Geometry check sheet. Reference: the model listing, model coordinates, mm. A direction names the side the tool comes from. Coordinates: 2 decimals unless noted, no trailing zeros. Write each loop counter-clockwise with the first axis right and the second up, starting at its lowest first coordinate (ties: lowest second). Pieces come first, ordered by that corner, then holes. Notation, with made-up numbers: M 77,-33 L 91,-33 A23 cw 91,-6 Z; hole C -39.75,-7.75 d3. An arc over 180 degrees is marked long. Put each result on its own line as item: value. Start each with the question number.
1) Gauge pin test, flat ends, axial feed: pin 1 (3 mm diameter, centred on x = 110.5, z = -85.5, fed in from -Y); pin 2 (6.5 mm diameter, centred on x = 89, z = -85, fed in from -Y). Record the tip position at first contact, or that the pin passes through.
2) Cross-section at B-B on z = -85. Record the cut outline in (x, y).
3) Cross-section at A-A on x = 111. Record the cut outline in (y, z).
4) Mould release check, pull along X, two halves, no side actions. Record for faces 1 (the flat face through (99, 5, -100)), 2 (the flat face through (200, 5, -49)), 3 (the flat face through (108, 3.3, -85)): released by +X, released by -X, zero draft, split by the parting line, or undercut.
5) Set-up check for faces 4 (the flat face through (99, 0, -51)), 5 (the cylindrical face through (106.363, 1.627, -83.97)): record each of +Z, -Z, +X, -X, +Y, -Y from which the full face is reachable in a straight line by a thin tool's end or side.
6) Scan lines: line 1 along X through (y, z) = (5, -85); line 2 along X through (y, z) = (2.5, -85). Record each from-to range of solid material in increasing order.
from build123d import *

# Parameters (mm, degrees)
SKETCH_1_W                   = 200
SKETCH_1_H                   = 100
EXTRUDE_1_DEPTH              = 10
HOLE_WIZARD_M5_2_D           = 5.5
HOLE_WIZARD_M5_2_CBORE_D     = 9.5
HOLE_WIZARD_M5_2_CBORE_DEPTH = 3.3


with BuildPart() as part:
    # 스케치1 → 보스-돌출1 (new body)
    with BuildSketch(Plane(origin=(0, 0, 0), x_dir=(1, 0, 0), z_dir=(0, 1, 0))):
        with Locations((100, 50)):
            Rectangle(SKETCH_1_W, SKETCH_1_H)
    extrude(amount=EXTRUDE_1_DEPTH)

    # M5 치즈머리 홈붙이 머리용 카운터보어2 (through all)
    with Locations(Plane(origin=(89, 0, -45), x_dir=(0, 0, -1), z_dir=(0, -1, 0))):
        with Locations((0, 0), (0, 22), (40, 22), (40, 0)):
            CounterBoreHole(HOLE_WIZARD_M5_2_D / 2, HOLE_WIZARD_M5_2_CBORE_D / 2, HOLE_WIZARD_M5_2_CBORE_DEPTH)


solid = part.part
Answer key:
1. pin 1: passes through
1. pin 2: stops at y = 3.3
2. outline: M 0,0 L 84.25,0 L 84.25,3.3 L 86.25,3.3 L 86.25,10 L 0,10 Z; M 91.75,3.3 L 93.75,3.3 L 93.75,0 L 106.25,0 L 106.25,3.3 L 108.25,3.3 L 108.25,10 L 91.75,10 Z; M 113.75,3.3 L 115.75,3.3 L 115.75,0 L 200,0 L 200,10 L 113.75,10 Z
3. outline: M 0,-100 L 10,-100 L 10,-87.75 L 3.3,-87.75 L 3.3,-89.75 L 0,-89.75 Z; M 0,-80.25 L 3.3,-80.25 L 3.3,-82.25 L 10,-82.25 L 10,-47.75 L 3.3,-47.75 L 3.3,-49.75 L 0,-49.75 Z; M 0,-40.25 L 3.3,-40.25 L 3.3,-42.25 L 10,-42.25 L 10,0 L 0,0 Z
4. face 1: zero draft
4. face 2: released by +X
4. face 3: undercut
5. face 4: +Z, -Z, +X, -X, -Y
5. face 5: -Y
6. line 1: x = 0 to 86.25, 91.75 to 108.25, 113.75 to 200
6. line 2: x = 0 to 84.25, 93.75 to 106.25, 115.75 to 200
